Geometry: final body of the model. Coordinates: model frame, mm. A direction names the side the tool comes from. Round coordinates to 2 decimals unless told otherwise and drop trailing zeros. Answer in a Markdown table with one row per item. Add a question column.
from build123d import *

# Parameters (mm, degrees)
SKETCH1_W           = 600
SKETCH1_H           = 20
BOSS_EXTRUDE1_DEPTH = 800
CUT_EXTRUDE1_DEPTH  = 1001.199980004


with BuildPart() as part:
    # Sketch1 → Boss-Extrude1 (new body)
    with BuildSketch(Plane.XY):
        with Locations((-300, 10)):
            Rectangle(SKETCH1_W, SKETCH1_H)
    extrude(amount=BOSS_EXTRUDE1_DEPTH)

    # Sketch2 → Cut-Extrude1 (cut, through all)
    with BuildSketch(Plane.XY.offset(800)):
        Polygon((-580, 20), (-580, 13.5), (-583, 13.5), (-583, 5.5), (-567, 5.5), (-567, 13.5), (-570, 13.5), (-570, 20), align=None)
        Polygon((-530, 20), (-530, 13.5), (-533, 13.5), (-533, 5.5), (-517, 5.5), (-517, 13.5), (-520, 13.5), (-520, 20), align=None)
        Polygon((-480, 20), (-480, 13.5), (-483, 13.5), (-483, 5.5), (-467, 5.5), (-467, 13.5), (-470, 13.5), (-470, 20), align=None)
        Polygon((-430, 20), (-430, 13.5), (-433, 13.5), (-433, 5.5), (-417, 5.5), (-417, 13.5), (-420, 13.5), (-420, 20), align=None)
        Polygon((-380, 20), (-380, 13.5), (-383, 13.5), (-383, 5.5), (-367, 5.5), (-367, 13.5), (-370, 13.5), (-370, 20), align=None)
        Polygon((-330, 20), (-330, 13.5), (-333, 13.5), (-333, 5.5), (-317, 5.5), (-317, 13.5), (-320, 13.5), (-320, 20), align=None)
        Polygon((-280, 20), (-280, 13.5), (-283, 13.5), (-283, 5.5), (-267, 5.5), (-267, 13.5), (-270, 13.5), (-270, 20), align=None)
        Polygon((-230, 20), (-230, 13.5), (-233, 13.5), (-233, 5.5), (-217, 5.5), (-217, 13.5), (-220, 13.5), (-220, 20), align=None)
        Polygon((-180, 20), (-180, 13.5), (-183, 13.5), (-183, 5.5), (-167, 5.5), (-167, 13.5), (-170, 13.5), (-170, 20), align=None)
        Polygon((-130, 20), (-130, 13.5), (-133, 13.5), (-133, 5.5), (-117, 5.5), (-117, 13.5), (-120, 13.5), (-120, 20), align=None)
        Polygon((-80, 20), (-80, 13.5), (-83, 13.5), (-83, 5.5), (-67, 5.5), (-67, 13.5), (-70, 13.5), (-70, 20), align=None)
        Polygon((-30, 20), (-30, 13.5), (-33, 13.5), (-33, 5.5), (-17, 5.5), (-17, 13.5), (-20, 13.5), (-20, 20), align=None)
    extrude(amount=-CUT_EXTRUDE1_DEPTH, mode=Mode.SUBTRACT)


solid = part.part
1) Section A-A, the plane y = 16.5. Give the number of separate pieces and of enclosed holes in the cut face, and give its area (3 significant figures).
2) Material intervals for line 1 along Y through (x, z) = (-382.5, 272); line 2 along Y through (x, z) = (-74.5, 313), sorted ascending. Write a range as from..to.
3) Pull-direction query (X, two-part tool) for faces 3 (the flat face through (-150, 20, 394)), 4 (the flat face through (-475, 5.5, 406)); classes: pulls with the +X half, pulls with the -X half, needs draft (parallel to the pull), parting line crosses it, or undercut.
4) Reachability of faces 1 (the flat face through (-200, 20, 394)), 2 (the flat face through (-575, 5.5, 406)) from +Z, -Z, +X, -X, +Y, -Y: full face, straight path, thin tool, end or side. Return the list, or none.
Evaluation:
| question | item | result |
|---|---|---|
| 1 | separate pieces | 13 |
| 1 | enclosed holes | 0 |
| 1 | area | 384,000 mm² |
| 2 | line 1 | y = 0..5.5, 13.5..20 |
| 2 | line 2 | y = 0..5.5 |
| 3 | face 3 | needs draft |
| 3 | face 4 | undercut |
| 4 | face 1 | +Z, -Z, +X, -X, +Y |
| 4 | face 2 | +Z, -Z |
